Verification items for this drawing (mm, ordinates from the low corner). Coordinates: 2 decimals unless noted, no trailing zeros. Write each loop counter-clockwise with the first axis right and the second up, starting at its lowest first coordinate (ties: lowest second). Pieces come first, ordered by that corner, then holes. Notation, with made-up numbers: (43.25, -8) -> (75.25, -8) arc R11 ccw to (75.25, 4) -> close; hole circle Ø10 at (26, 46.25). An arc over 180 degrees is marked (long way). Answer as CSV lines item,"result".
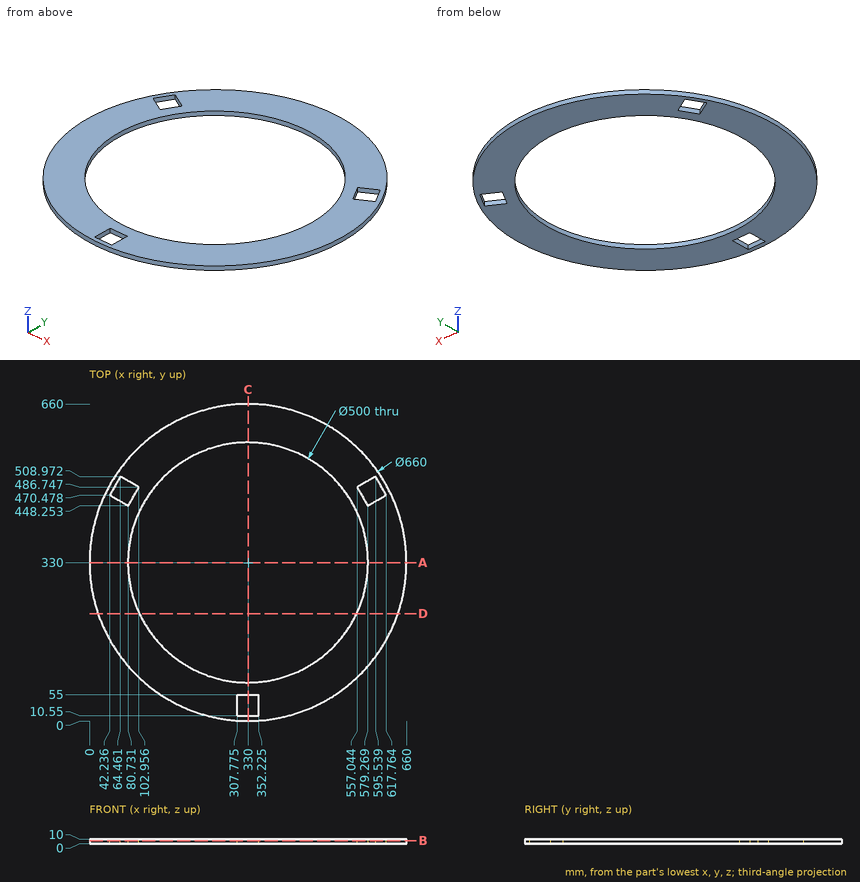
Item 1: Cross-section at A-A, the plane y = 330. Record the cut outline in (x, z), plus the area to 3 significant figures.
Responses:
outline,"(0, 0) -> (80, 0) -> (80, 10) -> (0, 10) -> close; (580, 0) -> (660, 0) -> (660, 10) -> (580, 10) -> close"
area,"1,600 mm2"
Item 2: Depth check by flat-ended pin: pin 1 Ø3 at (y, z) = (35, 2.5) entering from -X (1 decimal); pin 2 Ø6 at (y, z) = (299.5, 4.5) entering from -X; pin 3 Ø1 at (y, z) = (432, 2) entering from -X; pin 4 Ø1.5 at (x, y) = (83, 314) entering from -Z. Enter the tip coordinate at first touch or a pass-through.
Responses:
pin 1,"stops at x = 179.1"
pin 2,"stops at x = 1.15"
pin 3,"stops at x = 16"
pin 4,"passes through"
Item 3: Cross-section at D-D, the plane y = 223.5. Record the cut outline in (x, z), plus the area to 3 significant figures.
Responses:
outline,"(17.66, 0) -> (103.82, 0) -> (103.82, 10) -> (17.66, 10) -> close; (556.18, 0) -> (642.34, 0) -> (642.34, 10) -> (556.18, 10) -> close"
area,"1,720 mm2"
Item 4: Cross-section at C-C, the plane x = 330. Record the cut outline in (y, z).
Responses:
outline,"(0, 0) -> (10.55, 0) -> (10.55, 10) -> (0, 10) -> close; (55, 0) -> (80, 0) -> (80, 10) -> (55, 10) -> close; (580, 0) -> (660, 0) -> (660, 10) -> (580, 10) -> close"
Item 5: Cross-section at B-B, the plane z = 6.5. Count the separate pieces of the cut face and the enclosed holes in it, plus the area to 3 significant figures.
Responses:
separate pieces,"1"
enclosed holes,"4"
area,"140,000 mm2"
Item 6: Thickness scan on probe 1 along Y at (x, z) = (330, 8); probe 2 along X at (y, z) = (370, 9); probe 3 along Y at (x, z) = (180.5, 3.5) (1 decimal). Record the ranges inside material, lowest first.
Responses:
probe 1,"y = 0 to 10.55, 55 to 80, 580 to 660"
probe 2,"x = 2.43 to 83.22, 576.78 to 657.57"
probe 3,"y = 35.8 to 129.6, 530.4 to 624.2"
